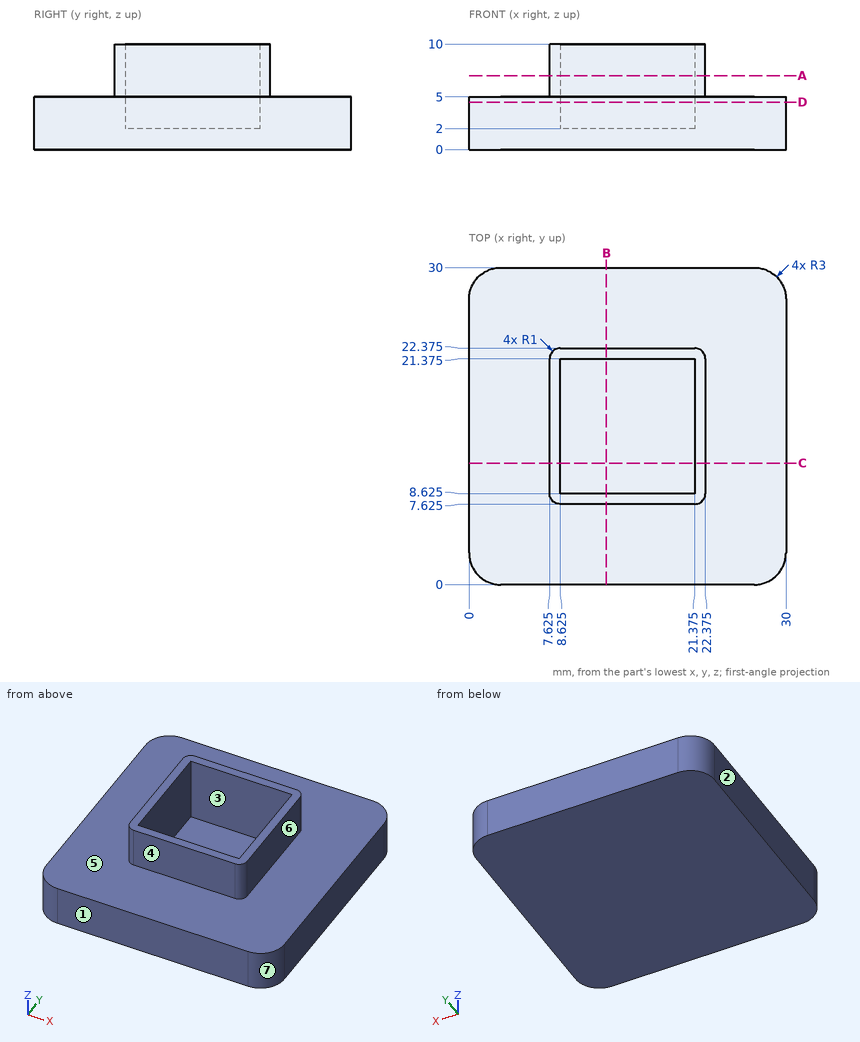
Geometry: see drawing. Coordinates: mm, zero at the bounding-box minimum. A direction names the side the tool comes from. Coordinates: 2 decimals unless noted, no trailing zeros. Loops run counter-clockwise (first coordinate to the right, second up) from the corner with the lowest first, then second, coordinate; pieces in that order, holes last. Notation, with made-up numbers: M 69,52.5 L 112,52.5 A31 ccw 112,83.5 Z; hole C 14.5,36 d7. An arc over 180 degrees is marked long. Answer in a Markdown table with one row per item.
1. Section A-A, the plane z = 7. Output: boundary loops of the cut face in (x, y) (3 decimals).
Response:
| item | result |
|---|---|
| outline | M 7.625,8.625 A1 ccw 8.625,7.625 L 21.375,7.625 A1 ccw 22.375,8.625 L 22.375,21.375 A1 ccw 21.375,22.375 L 8.625,22.375 A1 ccw 7.625,21.375 Z; hole M 8.625,8.625 L 21.375,8.625 L 21.375,21.375 L 8.625,21.375 Z |
2. Draft query along X for the marked faces 1, 2 and 3. Return one class per face: pulls with the +X half, pulls with the -X half, needs draft (parallel to the pull), parting line crosses it, or undercut.
Response:
| item | result |
|---|---|
| face 1 | needs draft |
| face 2 | pulls with the -X half |
| face 3 | undercut |
3. Material intervals for line 1 (X direction, y = 20.25, z = 4) (3 decimals); line 2 (X direction, y = 12.75, z = 8.5) (3 decimals), sorted ascending.
Response:
| item | result |
|---|---|
| line 1 | x = 0 to 8.625, 21.375 to 30 |
| line 2 | x = 7.625 to 8.625, 21.375 to 22.375 |
4. First-contact query: pin 1 (6.5 mm diameter, centred on x = 17, y = 12.5, fed in from +Z); pin 2 (5.5 mm diameter, centred on x = 15.5, z = 8.5, fed in from +Y) (3 decimals); pin 3 (4 mm diameter, centred on y = 17.5, z = 8.5, fed in from -X) (3 decimals). Flat tips, straight axial feed; report the tip coordinate or a pass-through.
Response:
| item | result |
|---|---|
| pin 1 | stops at z = 2 |
| pin 2 | stops at y = 22.375 |
| pin 3 | stops at x = 7.625 |
5. Reachability of the marked faces 4, 5, 6 and 7 from +Z, -Z, +X, -X, +Y, -Y: full face, straight path, thin tool, end or side. Return the list, or none.
Response:
| item | result |
|---|---|
| face 4 | +Z, +X, -X, -Y |
| face 5 | +Z |
| face 6 | +Z, +X, +Y, -Y |
| face 7 | +Z, -Z, +X, -Y |
6. Section B-B, the plane x = 13. Output: boundary loops of the cut face in (y, z) (3 decimals), then the cut area to 3 significant figures.
Response:
| item | result |
|---|---|
| outline | M 0,0 L 30,0 L 30,5 L 22.375,5 L 22.375,10 L 21.375,10 L 21.375,2 L 8.625,2 L 8.625,10 L 7.625,10 L 7.625,5 L 0,5 Z |
| area | 122 mm2 |
7. Section D-D, the plane z = 4.5. Output: boundary loops of the cut face in (x, y) (3 decimals), then the cut area to 3 significant figures.
Response:
| item | result |
|---|---|
| outline | M 0,3 A3 ccw 3,0 L 27,0 A3 ccw 30,3 L 30,27 A3 ccw 27,30 L 3,30 A3 ccw 0,27 Z; hole M 8.625,8.625 L 21.375,8.625 L 21.375,21.375 L 8.625,21.375 Z |
| area | 730 mm2 |
